Autodesk Inventor part; units mm, degrees
ref_plane "YZ Plane" through (0, 0, 0) normal (1, 0, 0) x (0, 1, 0)
ref_plane "XZ Plane" through (0, 0, 0) normal (0, 1, 0) x (-1, 0, 0)
ref_plane "XY Plane" through (0, 0, 0) normal (0, 0, 1) x (1, 0, 0)
sketch "Sketch1" plane through (0, 0, 0) normal (0, 1, 0) x (-1, 0, 0)
  circle A0 centre (0, 0) radius 3
  dimension "d0" = 6
extrude "Extrusion1" add sketch "Sketch1" against normal blind 3
sketch "Sketch2" plane through (0, -3, 0) normal (0, -1, 0) x (1, 0, 0)
  circle A0 centre (0, 0) radius 1.5
  dimension "d3" = 3
extrude "Extrusion2" add sketch "Sketch2" along normal blind 16
sketch "Sketch3" plane through (0, 0, 0) normal (0, 1, 0) x (1, 0, 0)
  circle A0 centre (0, 0) radius 1.5 construction
  line L0 (1.4434, 0) -> (0.7217, -1.25)
  line L1 (0.7217, -1.25) -> (-0.7217, -1.25)
  line L2 (-0.7217, -1.25) -> (-1.4434, 0)
  line L3 (-1.4434, 0) -> (-0.7217, 1.25)
  line L4 (-0.7217, 1.25) -> (0.7217, 1.25)
  line L5 (0.7217, 1.25) -> (1.4434, 0)
  dimension "d8" = 2.5
extrude "Extrusion3" cut sketch "Sketch3" against normal blind 1.5
chamfer "Chamfer1" distance 0.25 angle 45 1 edges at (-1.5, -19, 0)
fillet "Fillet1" radius 0.25 2 edges at (3, 0, 0) (3, -3, 0)
chamfer "Chamfer2" distance 0.1 angle 45 6 edges at (0, 0, -1.25) (1.0825, 0, -0.625) (1.0825, 0, 0.625) (0, 0, 1.25) (-1.0825, 0, 0.625) (-1.0825, 0, -0.625)
thread "Thread2"
properties part number "M3-16" material "Steel, Carbon"
The listing builds one solid part. Answer for the finished solid, in the listing's coordinates (mm). A direction names the side the tool comes from. Give positions to 0.01 mm unless a question says otherwise; leave off trailing zeros. Loops run counter-clockwise (first coordinate to the right, second up) from the corner with the lowest first, then second, coordinate; pieces in that order, holes last. Notation, with made-up numbers: (47, -19.75) - (70, -19.75) arc R30 ccw to (70, 12.25) - close; hole circle Ø3 at (30.5, 18). An arc over 180 degrees is marked (long way). Return JSON: item names as keys, results as strings. Group by question number.
1. Find section B-B (y = -13.75). Write down the section's boundary in (x, z), then the cut area to 3 significant figures.
2. Determine the mould class of faces 1 (the flat face through (-1.2, -3, -1.2)), 2 (the cylindrical face through (-1.5, -10.76, -0.07)), 3 (the flat face through (0, -1.5, 0)) for opening direction Z: pulls with the +Z half, pulls with the -Z half, needs draft (parallel to the pull), parting line crosses it, or undercut.
3. Which of the six approach directions +Z, -Z, +X, -X, +Y, -Y give full straight-line access (tool end or side, diameter ignored) to faces 4 (the flat face through (0, -1, -1.25)), 5 (the cylindrical face through (3, -1, 0))?
4. Straight lines are drawn through the part: line 1 (Y direction, x = -2.25, z = -1.25); line 2 (Z direction, x = 0, y = -4.5); line 3 (Y direction, x = 0, z = 0.75). For each, find the intervals that lie inside material, in ascending order. Write a range as [from, to].
5. Find section A-A (x = 0). Write down the section's boundary in (y, z).
Verdict:
{
 "1": {"outline": "circle Ø3 at (0, 0)", "area": "7.07 mm^2"},
 "2": {"face 1": "needs draft", "face 2": "parting line crosses it", "face 3": "undercut"},
 "3": {"face 4": "+Y", "face 5": "+Y, -Y"},
 "4": {"line 1": "y = [-3, 0]", "line 2": "z = [-1.5, 1.5]", "line 3": "y = [-19, -1.5]"},
 "5": {"outline": "(-19, -1.25) - (-18.75, -1.5) - (-3, -1.5) - (-3, -2.75) arc R0.25 ccw to (-2.75, -3) - (-0.25, -3) arc R0.25 ccw to (0, -2.75) - (0, -1.35) - (-0.1, -1.25) - (-1.5, -1.25) - (-1.5, 1.25) - (-0.1, 1.25) - (0, 1.35) - (0, 2.75) arc R0.25 ccw to (-0.25, 3) - (-2.75, 3) arc R0.25 ccw to (-3, 2.75) - (-3, 1.5) - (-18.75, 1.5) - (-19, 1.25) - close"}
}
